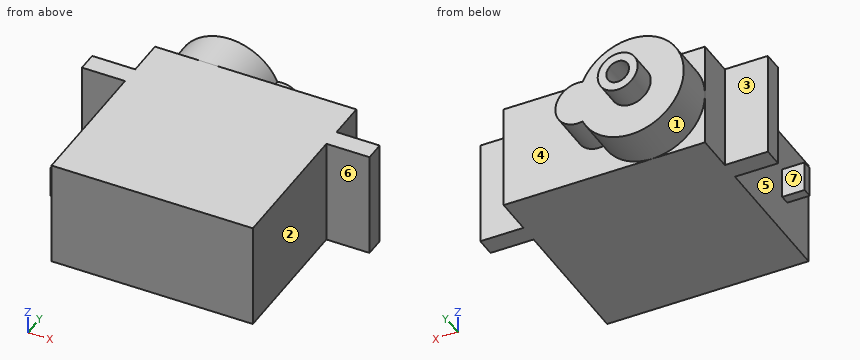
Autodesk Inventor part; units mm, degrees
ref_plane "YZ Plane" through (0, 0, 0) normal (1, 0, 0) x (0, 1, 0)
ref_plane "XZ Plane" through (0, 0, 0) normal (0, 1, 0) x (-1, 0, 0)
ref_plane "XY Plane" through (0, 0, 0) normal (0, 0, 1) x (1, 0, 0)
sketch "Sketch1" plane through (0, 0, 0) normal (0, 0, 1) x (1, 0, 0)
  line L0 (0, 0) -> (22.7838, 0)
  line L1 (22.7838, 0) -> (22.7838, 22.479)
  line L2 (22.7838, 22.479) -> (0, 22.479)
  line L3 (0, 22.479) -> (0, 0)
  dimension "d0" = 22.7838
  dimension "d1" = 22.479
extrude "Extrusion1" add sketch "Sketch1" along normal blind 11.9888
sketch "Sketch2" plane through (0, 0, 0) normal (-1, 0, 0) x (0, 0, 1)
  line L0 (0, 22.479) -> (11.9888, 22.479)
  line L1 (0, 22.479) -> (0, 0)
  line L2 (0, 0) -> (11.9888, 0)
  line L3 (11.9888, 22.479) -> (11.9888, 0)
  line L4 (0, 22.479) -> (11.9888, 22.479)
  line L5 (0, 0) -> (0, 22.479)
  line L6 (11.9888, 0) -> (11.9888, 22.479)
  line L7 (0, 18.1864) -> (11.9888, 18.1864)
  line L8 (11.9888, 18.1864) -> (11.9888, 15.9766)
  line L9 (11.9888, 15.9766) -> (0, 15.9766)
  line L10 (0, 15.9766) -> (0, 18.1864)
  dimension "d4" = 2.2098
  dimension "d5" = 4.2926
extrude "Extrusion2" add sketch "Sketch2" along normal blind 4.8768 and the other way blind 27.6606 contours L7 L3 L9 L1
sketch "Sketch3" plane through (0, 0, 0) normal (-1, 0, 0) x (0, 0, 1)
  line L0 (0, 15.9766) -> (0, 0)
  line L1 (0, 0) -> (11.9888, 0)
  line L2 (4.2672, 5.715) -> (7.7216, 5.715)
  line L3 (7.7216, 5.715) -> (7.7216, 4.6228)
  line L4 (7.7216, 4.6228) -> (4.2672, 4.6228)
  line L5 (4.2672, 4.6228) -> (4.2672, 5.715)
  dimension "d10" = 3.4544
  dimension "d11" = 1.0922
  dimension "d12" = 4.6228
  dimension "d13" = 4.2672
extrude "Extrusion3" add sketch "Sketch3" along normal blind 2.54
sketch "Sketch4" plane through (0, 22.479, 0) normal (0, 1, 0) x (1, 0, 0)
  line L0 (22.7838, 0) -> (0, 0)
  line L1 (0, 0) -> (0, -11.9888)
  line L2 (22.7838, -11.9888) -> (0, -11.9888)
  circle A0 centre (5.9944, -5.9944) radius 5.9944
  circle A1 centre (11.9888, -5.9944) radius 2.54
  dimension "d17" = 5.08
extrude "Extrusion4" add sketch "Sketch4" along normal blind 4.6228 contours A0 A1 | A1 A0 | A0 A1
sketch "Sketch5" plane through (0, 27.1018, 0) normal (0, 1, 0) x (1, 0, 0)
  arc A0 (11.4507, -3.5121) -> (11.4507, -8.4767) centre (5.9944, -5.9944) ccw
  circle A1 centre (5.9944, -5.9944) radius 2.2606
  circle A2 centre (5.9944, -5.9944) radius 1.2827
  point P0 (0, 0)
  dimension "d20" = 4.5212
  dimension "d21" = 2.5654
extrude "Extrusion5" add sketch "Sketch5" along normal blind 2.8448
properties part number "servo body"
Model file for the job. Use its own axes, mm. Face numbers are marked on the shaded views. A direction names the side the tool comes from. Give positions to 0.01 mm unless a question says otherwise; leave off trailing zeros. Loops run counter-clockwise (first coordinate to the right, second up) from the corner with the lowest first, then second, coordinate; pieces in that order, holes last.
1) Wall check: line 1 (X direction, y = 12.5, z = 8); line 2 (Y direction, x = 5, z = 2); line 3 (Y direction, x = -2, z = 7.25) (3 decimals). Give the ranges that are in metal, low to high.
2) Pull direction Y, two halves, no side cores. Call the marked faces 4, 5, 6 and 7: +Y half, -Y half, draft (parallel to the pull), parting line (faces both ways), or undercut.
3) Saw through at A-A (z = 5.25). Write the cut outline in (x, y) (3 decimals), plus the area to 3 significant figures.
4) Saw through at B-B (x = 12). Write the cut outline in (y, z).
5) Saw through at D-D (x = 15.5). Write the cut outline in (y, z), plus the area to 3 significant figures.
6) Saw through at C-C (y = 19.75). Write the cut outline in (x, z), plus the area to 3 significant figures.
7) Flat gauge pins, fed straight in: pin 1 Ø1.5 at (x, z) = (24.5, 5.5) entering from -Y; pin 2 Ø0.9 at (y, z) = (5.5, 5.5) entering from -X; pin 3 Ø1.2 at (x, y) = (-1.5, 5.5) entering from +Z. Where does each tip first touch, or does it go through?
8) Tool access for the marked faces 1, 2 and 3: list every direction of +Z, -Z, +X, -X, +Y, -Y with a clear straight run to the whole face (end or side of a thin tool).
Answer block:
1. line 1: x = 0 to 22.78
1. line 2: y = 0 to 27.1
1. line 3: y = 4.623 to 5.715, 15.977 to 18.186
2. face 4: +Y half
2. face 5: undercut
2. face 6: -Y half
2. face 7: undercut
3. outline: (-4.877, 15.977) - (0, 15.977) - (0, 5.715) - (-2.54, 5.715) - (-2.54, 4.623) - (0, 4.623) - (0, 0) - (22.784, 0) - (22.784, 15.977) - (27.661, 15.977) - (27.661, 18.186) - (22.784, 18.186) - (22.784, 22.479) - (14.417, 22.479) - (14.417, 27.102) - (8.129, 27.102) - (8.129, 29.947) - (7.039, 29.947) - (7.039, 27.102) - (4.95, 27.102) - (4.95, 29.947) - (3.86, 29.947) - (3.86, 27.102) - (0.046, 27.102) - (0.046, 22.479) - (0, 22.479) - (0, 18.186) - (-4.877, 18.186) - close
3. area: 609 mm2
4. outline: (0, 0) - (22.48, 0) - (22.48, 3.45) - (27.1, 3.45) - (27.1, 8.53) - (22.48, 8.53) - (22.48, 11.99) - (0, 11.99) - close
5. outline: (0, 0) - (22.48, 0) - (22.48, 11.99) - (0, 11.99) - close
5. area: 269 mm2
6. outline: (0, 0) - (22.78, 0) - (22.78, 11.99) - (0, 11.99) - close
6. area: 273 mm2
7. pin 1: stops at y = 15.98
7. pin 2: stops at x = -2.54
7. pin 3: stops at z = 7.72
8. face 1: +Y
8. face 2: +Z, -Z, +X, -Y
8. face 3: +Z, -Z, -X, +Y
